```python
from build123d import *

# Parameters (mm, degrees)
SKETCH1_R           = 30.5
BOSS_EXTRUDE1_DEPTH = 15
SKETCH2_R           = 3.5
CUT_EXTRUDE1_DEPTH  = 15
SKETCH3_R           = 20
BOSS_EXTRUDE2_DEPTH = 65
SKETCH4_R           = 12.5
BOSS_EXTRUDE3_DEPTH = 42.7
CUT_EXTRUDE2_START  = -10.675
SKETCH5_R           = 12.5
SKETCH5_R_2         = 6.25
CUT_EXTRUDE2_DEPTH  = 10.675
FILLET1_R           = 6.25
CHAMFER1_SIZE       = 6.25


with BuildPart() as part:
    # Sketch1 → Boss-Extrude1 (new body)
    with BuildSketch(Plane.XY):
        Circle(SKETCH1_R)
    extrude(amount=BOSS_EXTRUDE1_DEPTH)

    # Sketch2 → Cut-Extrude1 (cut)
    with BuildSketch(Plane.XY.offset(15)):
        with Locations((0, 25)):
            Circle(SKETCH2_R)
        with Locations((25, 0)):
            Circle(SKETCH2_R)
        with Locations((0, -25)):
            Circle(SKETCH2_R)
        with Locations((-25, 0)):
            Circle(SKETCH2_R)
    extrude(amount=-CUT_EXTRUDE1_DEPTH, mode=Mode.SUBTRACT)

    # Sketch3 → Boss-Extrude2 (add)
    with BuildSketch(Plane.XY.offset(15)):
        Circle(SKETCH3_R)
    extrude(amount=BOSS_EXTRUDE2_DEPTH)

    # Sketch4 → Boss-Extrude3 (add)
    with BuildSketch(Plane.XY.offset(80)):
        with Locations(Location((0, 0, 0), (0, 0, 180))):
            Circle(SKETCH4_R)
    extrude(amount=BOSS_EXTRUDE3_DEPTH)

    # Sketch5 → Cut-Extrude2 (cut)
    with BuildSketch(Plane.XY.offset(122.7).offset(CUT_EXTRUDE2_START)):
        with Locations(Location((0, 0, 0), (0, 0, 180))):
            Circle(SKETCH5_R)
        Circle(SKETCH5_R_2, mode=Mode.SUBTRACT)
    extrude(amount=CUT_EXTRUDE2_DEPTH, mode=Mode.SUBTRACT)

    # Fillet1
    fillet1_edges = [part.edges().sort_by_distance(p)[0] for p in [
        (12.5, 0, 112.025),
    ]]
    fillet(fillet1_edges, radius=FILLET1_R - 0.0001)  # a hair under: the kernel refuses the full size

    # Chamfer1
    chamfer1_edges = [part.edges().sort_by_distance(p)[0] for p in [
        (-6.25, 0, 122.7),
    ]]
    chamfer(chamfer1_edges, length=CHAMFER1_SIZE)


solid = part.part
```
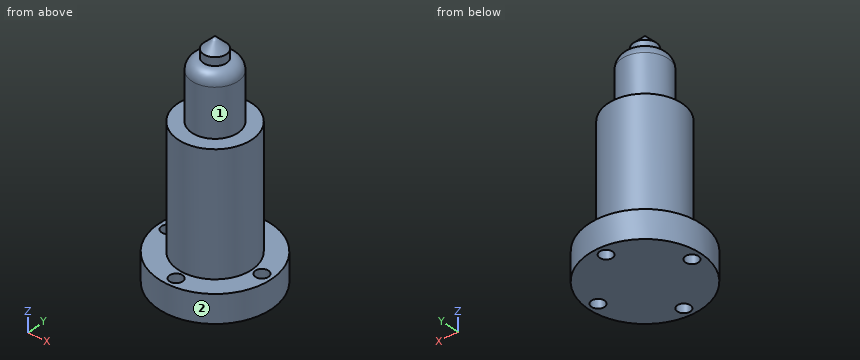
Input: part model. Units: mm. Frame: model coordinates. Face numbers are marked on the shaded views. A direction names the side the tool comes from. Give positions to 0.01 mm unless a question says otherwise; leave off trailing zeros. Write each loop counter-clockwise with the first axis right and the second up, starting at its lowest first coordinate (ties: lowest second). Pieces come first, ordered by that corner, then holes. Notation, with made-up numbers: (29.5, -10.5) - (73.5, -10.5) arc R25 ccw to (73.5, 19.5) - close; hole circle Ø2 at (9, -24). An arc over 180 degrees is marked (long way). Write item = value, one per line. Start each with the question number.
1) Cut plane A-A (y = -26.5). Return loops of the section in (x, z).
2) Pin query (flat end, axial travel): pin 1 (6 mm diameter, centred on y = 10.5, z = 57.5, fed in from -X); pin 2 (2 mm diameter, centred on x = 19.5, z = 29.5, fed in from +Y); pin 3 (1.5 mm diameter, centred on x = -19.5, y = 7.5, fed in from +Z); pin 4 (6.5 mm diameter, centred on x = 25, y = 0, fed in from +Z). Return the tip coordinate at first contact, or that it passes through.
3) Reachability of the marked faces 1 and 2 from +Z, -Z, +X, -X, +Y, -Y: full face, straight path, thin tool, end or side. Return the list, or none.
4) Cut plane B-B (z = 46). Return loops of the section in (x, y), and give its area (3 significant figures).
5) Cut plane C-C (y = 23). Return loops of the section in (x, z), and give its area (3 significant figures).
6) Material intervals for L1, parallel to Y at x = 0, z = 9; L2, parallel to Z at x = 6, y = 22; L3, parallel to Z at x = -13.5, y = -5.5, sorted ascending. Write a range as [from, to].
7) Cut plane D-D (z = 110). Return loops of the section in (x, y), and give its area (3 significant figures).
Answers follow:
q1.outline = (-15.1, 0) - (-3.16, 0) - (-3.16, 15) - (-15.1, 15) - close; (3.16, 0) - (15.1, 0) - (15.1, 15) - (3.16, 15) - close
q2.pin_1 = -18.54
q2.pin_2 = 7.6
q2.pin_3 = 15
q2.pin_4 = through
q3.face_1 = +Z
q3.face_2 = +Z, -Z
q4.outline = circle Ø40 at (0, 0)
q4.area = 1,260 mm^2
q5.outline = (-20.03, 0) - (-2.87, 0) - (-2.87, 15) - (-20.03, 15) - close; (2.87, 0) - (20.03, 0) - (20.03, 15) - (2.87, 15) - close
q5.area = 515 mm^2
q6.L1 = [-30.5, -28.5], [-21.5, 21.5], [28.5, 30.5]
q6.L2 = [0, 15]
q6.L3 = [0, 80]
q7.outline = circle Ø21.71 at (0, 0)
q7.area = 370 mm^2
